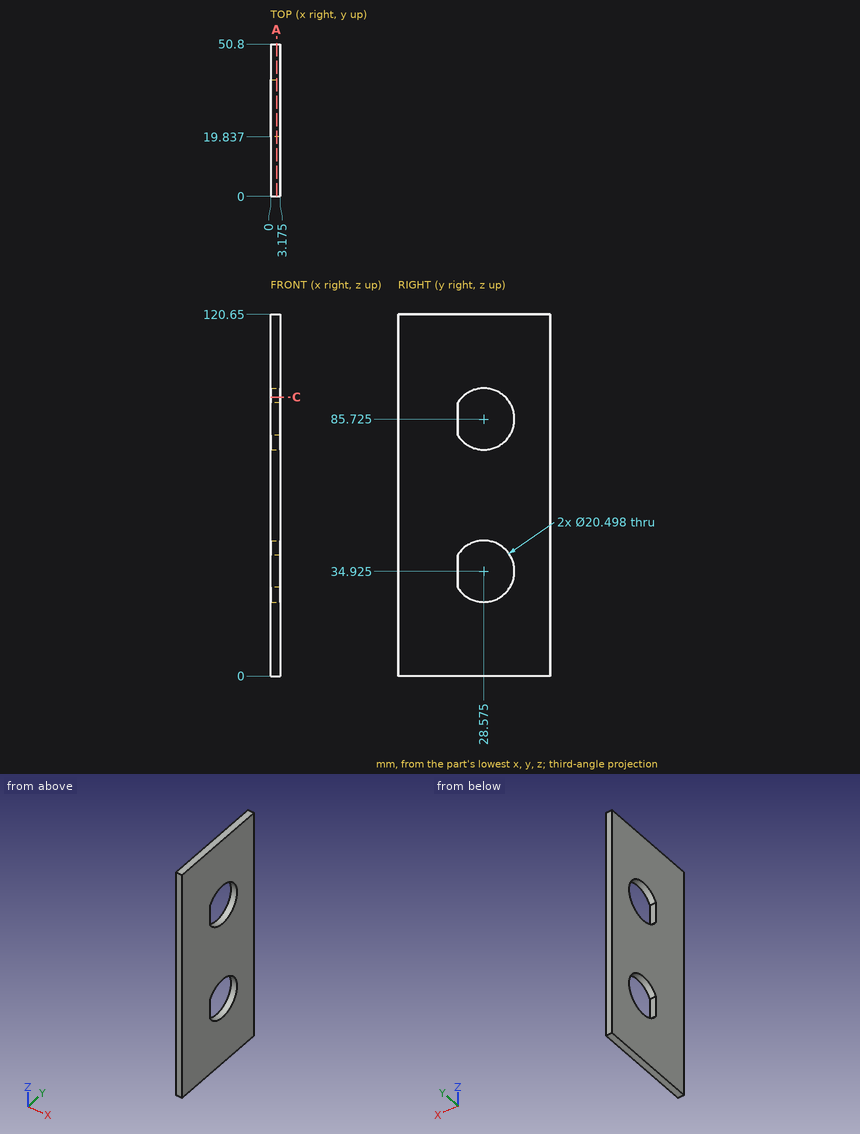
Design review of the part shown in the three views and the two pictorial views. Dimensions are in mm from the part's minimum x, y and z. Round coordinates to 2 decimals unless told otherwise and drop trailing zeros. Order: outer loops, then holes, each group sorted by start corner. A loop starts at its lowest first (then second) coordinate and runs counter-clockwise, first axis right, second up.
Item 1: Add section A-A, the plane x = 2.05. Count the separate pieces of the cut face and the enclosed holes in it, and give its area (3 significant figures).
Working result:
separate pieces: 1
enclosed holes: 2
area: 5,490 mm2
Item 2: To check wall thickness, follow probe 1 along Z at (x, y) = (1.6, 37); probe 2 along Y at (x, z) = (1.9, 28); probe 3 along Y at (x, z) = (1.8, 91.5). State the ranges of each line that lie inside material, in increasing order.
Working result:
probe 1: z = 0 to 29.09, 40.76 to 79.89, 91.56 to 120.65
probe 2: y = 0 to 21.02, 36.13 to 50.8
probe 3: y = 0 to 20.11, 37.04 to 50.8
Item 3: Add section C-C, the plane z = 93. State the section outline as (x, y) points (1 decimal).
Working result:
outline: (0, 0) - (3.2, 0) - (3.2, 21.4) - (0, 21.4) - close; (0, 35.8) - (3.2, 35.8) - (3.2, 50.8) - (0, 50.8) - close
